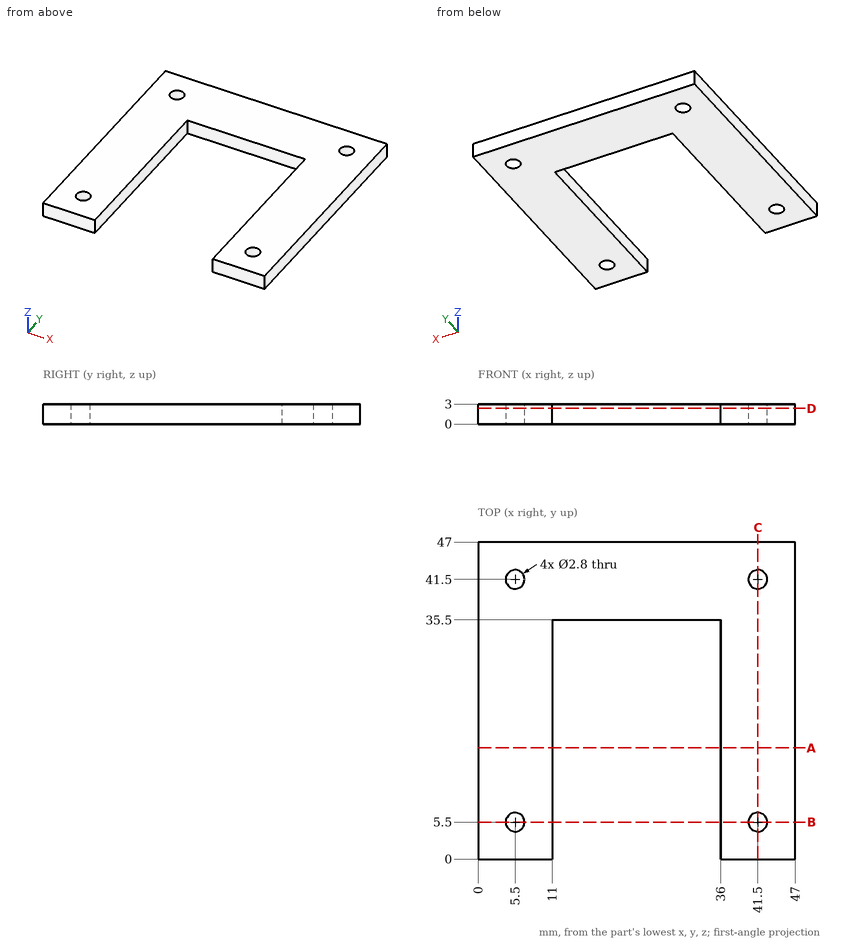
Part print with two shaded views. Sizes in mm from the minimum x, y, z corner. Give positions to 0.01 mm unless a question says otherwise; leave off trailing zeros. Order: outer loops, then holes, each group sorted by start corner. A loop starts at its lowest first (then second) coordinate and runs counter-clockwise, first axis right, second up.
1) Saw through at D-D, the plane z = 2.35. Write the cut outline in (x, y).
2) Saw through at A-A, the plane y = 16.5. Write the cut outline in (x, z).
3) Saw through at C-C, the plane x = 41.5. Write the cut outline in (y, z).
4) Saw through at B-B, the plane y = 5.5. Write the cut outline in (x, z).
5) Wall check: probe 1 along Y at (x, z) = (5.5, 2); probe 2 along Y at (x, z) = (41, 0.3); probe 3 along X at (y, z) = (9, 1.3). Give the ranges that are in metal, low to high.
Computed:
1. outline: (0, 0) - (11, 0) - (11, 35.5) - (36, 35.5) - (36, 0) - (47, 0) - (47, 47) - (0, 47) - close; hole circle Ø2.8 at (5.5, 5.5); hole circle Ø2.8 at (5.5, 41.5); hole circle Ø2.8 at (41.5, 5.5); hole circle Ø2.8 at (41.5, 41.5)
2. outline: (0, 0) - (11, 0) - (11, 3) - (0, 3) - close; (36, 0) - (47, 0) - (47, 3) - (36, 3) - close
3. outline: (0, 0) - (4.1, 0) - (4.1, 3) - (0, 3) - close; (6.9, 0) - (40.1, 0) - (40.1, 3) - (6.9, 3) - close; (42.9, 0) - (47, 0) - (47, 3) - (42.9, 3) - close
4. outline: (0, 0) - (4.1, 0) - (4.1, 3) - (0, 3) - close; (6.9, 0) - (11, 0) - (11, 3) - (6.9, 3) - close; (36, 0) - (40.1, 0) - (40.1, 3) - (36, 3) - close; (42.9, 0) - (47, 0) - (47, 3) - (42.9, 3) - close
5. probe 1: y = 0 to 4.1, 6.9 to 40.1, 42.9 to 47
5. probe 2: y = 0 to 4.19, 6.81 to 40.19, 42.81 to 47
5. probe 3: x = 0 to 11, 36 to 47
